Read the model definition and answer for the solid it produces. Units are mm, in the model's axes. Coordinates: 2 decimals unless noted, no trailing zeros. Loops run counter-clockwise (first coordinate to the right, second up) from the corner with the lowest first, then second, coordinate; pieces in that order, holes last.
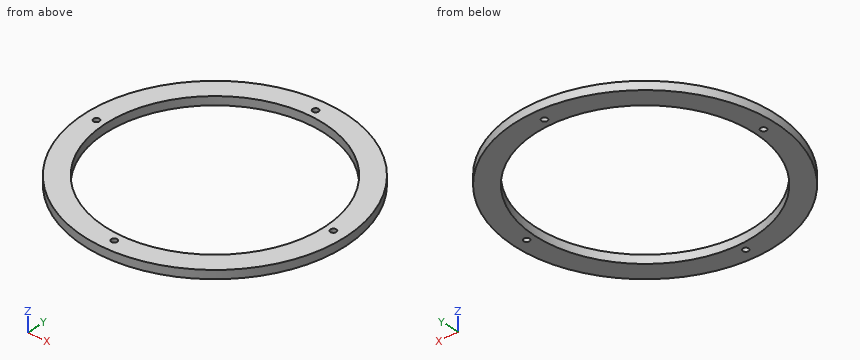
Autodesk Inventor part; units mm, degrees
ref_plane "YZ Plane" through (0, 0, 0) normal (1, 0, 0) x (0, 1, 0)
ref_plane "XZ Plane" through (0, 0, 0) normal (0, 1, 0) x (-1, 0, 0)
ref_plane "XY Plane" through (0, 0, 0) normal (0, 0, 1) x (1, 0, 0)
sketch "스케치1" plane through (0, 0, 0) normal (0, 0, 1) x (1, 0, 0)
  circle A0 centre (0, 0) radius 77.5
  circle A1 centre (0, 0) radius 65
  dimension "d0" = 155
  dimension "d1" = 130
extrude "돌출1" add sketch "스케치1" along normal blind 5
sketch "스케치2" plane through (0, 0, 5) normal (0, 0, 1) x (1, 0, 0)
  circle A0 centre (0, 70) radius 1.75
  circle A1 centre (-70, 0) radius 1.75
  circle A2 centre (0, -70) radius 1.75
  circle A3 centre (70, 0) radius 1.75
  point P0 (0, 0)
  dimension "d4" = 3.5
  dimension "d5" = 70
  dimension "d8" = 360
extrude "돌출2" cut sketch "스케치2" against normal blind 5
properties part number "아크릴 고정판"
Q1. Straight lines are drawn through the part: probe 1 along Y at (x, z) = (0, 3.3); probe 2 along X at (y, z) = (-11.5, 4.7); probe 3 along Y at (x, z) = (8, 3.85). For each, find the intervals that lie inside material, in ascending order.
Findings below:
probe 1: y = -77.5 to -71.75, -68.25 to -65, 65 to 68.25, 71.75 to 77.5
probe 2: x = -76.64 to -63.97, 63.97 to 76.64
probe 3: y = -77.09 to -64.51, 64.51 to 77.09
Q2. Flat-ended cylindrical pins translate along their axes: pin 1 Ø3 at (x, y) = (0, 70) entering from +Z; pin 2 Ø1.5 at (x, z) = (1.5, 4) entering from -Y; pin 3 Ø1.5 at (x, z) = (-8.5, 3) entering from -Y; pin 4 Ø4 at (x, y) = (70, 0) entering from +Z. Find the tip coordinate at first contact, or state that the pin passes through.
Findings below:
pin 1: passes through
pin 2: stops at y = -77.5
pin 3: stops at y = -77.11
pin 4: stops at z = 5
Q3. A cutting plane is placed at B-B (y = 46). Give the vertices of the cut face in (x, z), then the cut area to 3 significant figures.
Findings below:
outline: (-62.37, 0) - (-45.92, 0) - (-45.92, 5) - (-62.37, 5) - close; (45.92, 0) - (62.37, 0) - (62.37, 5) - (45.92, 5) - close
area: 164 mm2
Q4. A cutting plane is placed at A-A (x = -22). Give the vertices of the cut face in (y, z).
Findings below:
outline: (-74.31, 0) - (-61.16, 0) - (-61.16, 5) - (-74.31, 5) - close; (61.16, 0) - (74.31, 0) - (74.31, 5) - (61.16, 5) - close
Q5. A cutting plane is placed at C-C (z = 4.25). Give the vertices of the cut face in (x, y).
Findings below:
outline: circle Ø155 at (0, 0); hole circle Ø3.5 at (-70, 0); hole circle Ø130 at (0, 0); hole circle Ø3.5 at (0, -70); hole circle Ø3.5 at (0, 70); hole circle Ø3.5 at (70, 0)
